Input: part model. Units: mm. Frame: model coordinates. Face numbers are marked on the shaded views. Give positions to 0.01 mm unless a question says otherwise; leave off trailing zeros. Loops run counter-clockwise (first coordinate to the right, second up) from the corner with the lowest first, then second, coordinate; pieces in that order, holes last. Notation, with made-up numbers: M 75.5,81 L 106.5,81 A23 ccw 106.5,89 Z; hole C 58,70.5 d7. An arc over 180 degrees is marked long. One line per item, written item: value. Start each with the question number.
(1) Section A-A on x = -40. Output: boundary loops of the cut face in (y, z).
(2) Section D-D on x = -26.5. Output: boundary loops of the cut face in (y, z).
(3) Section B-B on y = -28. Output: boundary loops of the cut face in (x, z).
(4) Pin query (flat end, axial travel): P1, Ø3.5, axis at x = -40, y = -36, coming from the +Z side. Return the tip coordinate at first contact, or that it passes through.
(5) Pull-direction query (Y, two-part tool) for the marked faces 1, 2 and 3; classes: released by +Y, released by -Y, zero draft, split by the parting line, or undercut.
(6) Ray query, line 1 along Y through (x, z) = (-40, 67.8); line 2 along Y through (x, z) = (-20, 67.45); line 3 along Y through (x, z) = (-37.25, 66.8). Return the intervals inside material, ascending. Write a range as from..to.
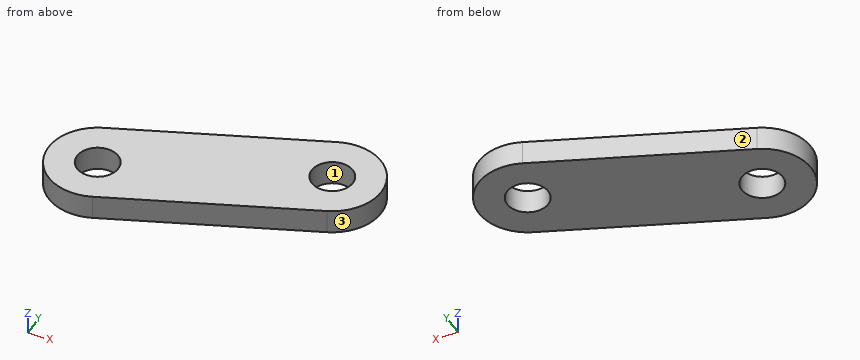
```python
from build123d import *

# Parameters (mm, degrees)
SK_BIELA_EXTERIOR_R  = 2.1
BIELA_EXTERIOR_DEPTH = 2.5


with BuildPart() as part:
    # Sk_Biela_exterior → Biela_exterior (new body)
    with BuildSketch(Plane.XY.offset(66.4)):
        with BuildLine():
            Line((-38.143046618, -40.642383454), (-18.143046618, -32.642383454))
            ThreePointArc((-18.143046618, -32.642383454), (-15.357616546, -26.143046618), (-21.856953382, -23.357616546))
            Line((-21.856953382, -23.357616546), (-41.856953382, -31.357616546))
            ThreePointArc((-41.856953382, -31.357616546), (-44.642383454, -37.856953382), (-38.143046618, -40.642383454))
        make_face()
        with Locations((-20, -28)):
            Circle(SK_BIELA_EXTERIOR_R, mode=Mode.SUBTRACT)
        with Locations((-40, -36)):
            Circle(SK_BIELA_EXTERIOR_R, mode=Mode.SUBTRACT)
    extrude(amount=BIELA_EXTERIOR_DEPTH)


solid = part.part
```
Output values:
1. outline: M -41,66.4 L -38.1,66.4 L -38.1,68.9 L -41,68.9 Z; M -33.9,66.4 L -30.61,66.4 L -30.61,68.9 L -33.9,68.9 Z
2. outline: M -35.99,66.4 L -25.21,66.4 L -25.21,68.9 L -35.99,68.9 Z
3. outline: M -33.46,66.4 L -22.1,66.4 L -22.1,68.9 L -33.46,68.9 Z; M -17.9,66.4 L -15,66.4 L -15,68.9 L -17.9,68.9 Z
4. P1: passes through
5. face 1: undercut
5. face 2: released by +Y
5. face 3: split by the parting line
6. line 1: y = -41..-38.1, -33.9..-30.61
6. line 2: y = -33.39..-30.1, -25.9..-23
6. line 3: y = -40.29..-29.51
